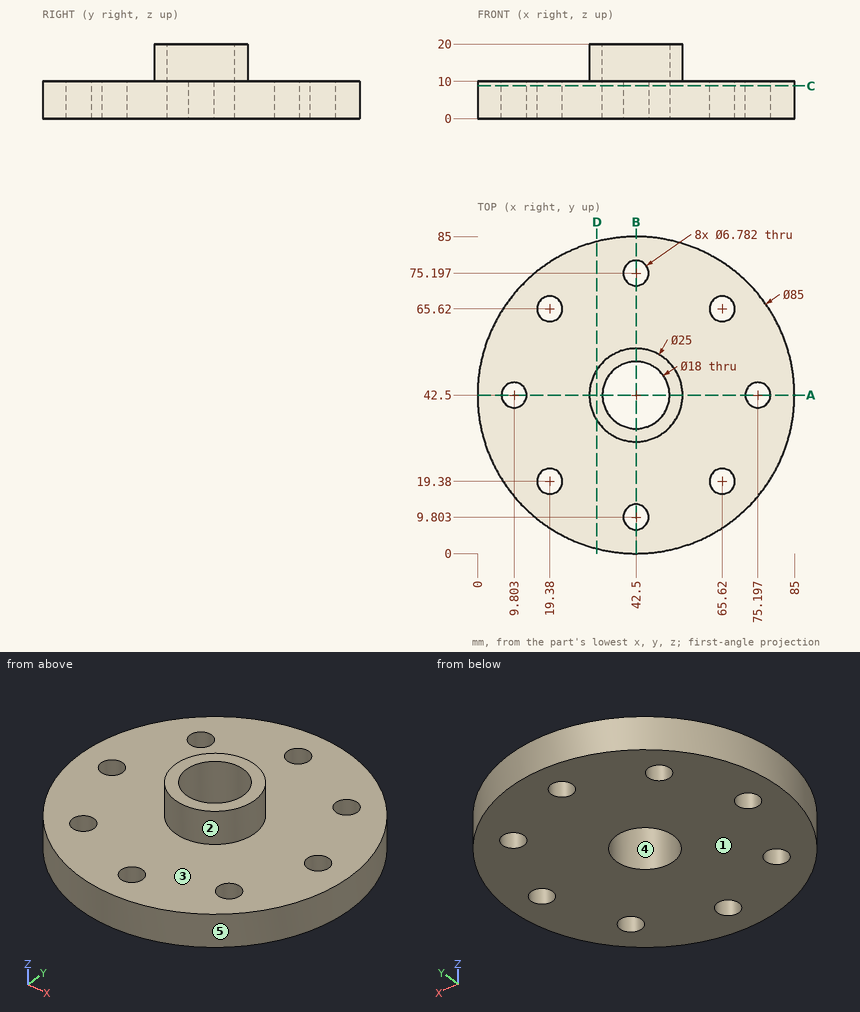
The figure shows three views and two pictorial views of one solid part (mm, origin at its lowest corner). Answer the questions. A direction names the side the tool comes from. Coordinates: 2 decimals unless noted, no trailing zeros. Loops run counter-clockwise (first coordinate to the right, second up) from the corner with the lowest first, then second, coordinate; pieces in that order, holes last. Notation, with made-up numbers: (-29.5, -1) -> (6.5, -1) arc R16 cw to (6.5, 23) -> close; hole circle Ø2 at (85, 23). An arc over 180 degrees is marked (long way). Return JSON: item names as keys, results as strings. Group by question number.
(1) Given pin 1 Ø5 at (x, y) = (16.5, 53.5) entering from +Z; pin 2 Ø1 at (x, z) = (37, 12) entering from -Y; pin 3 Ø10 at (x, z) = (75.5, 10) entering from +Y; pin 4 Ø4 at (x, y) = (19.38, 19.38) entering from -Z, each flat-ended and moving along its own axis, determine where each tip first touches the part or whether it passes through.
(2) A cutting plane is placed at D-D on x = 32. Write down the section's boundary in (y, z), and give its area (3 significant figures).
(3) Which of the six approach directions +Z, -Z, +X, -X, +Y, -Y give full straight-line access (tool end or side, diameter ignored) to the marked faces 1 and 2?
(4) A cutting plane is placed at A-A on y = 42.5. Write down the section's boundary in (x, z) (1 decimal).
(5) Find the intervals of material crossed by probe 1 along Y at (x, z) = (18, 7); probe 2 along Z at (x, y) = (16.5, 52); probe 3 along X at (y, z) = (41.5, 13.5) (1 decimal), in increasing order. Write a range as from..to.
(6) Determine the mould class of the marked faces 3, 4 and 5 for opening direction Y: released by +Y, released by -Y, zero draft, split by the parting line, or undercut.
(7) A cutting plane is placed at C-C on z = 8.75. Count the separate pieces of the cut face and the enclosed holes in it, and give its area (3 significant figures).
The answers:
{
 "1": {"pin 1": "stops at z = 10", "pin 2": "stops at y = 31.04", "pin 3": "stops at y = 74.47", "pin 4": "passes through"},
 "2": {"outline": "(1.32, 0) -> (83.68, 0) -> (83.68, 10) -> (49.28, 10) -> (49.28, 20) -> (35.72, 20) -> (35.72, 10) -> (1.32, 10) -> close", "area": "959 mm^2"},
 "3": {"face 1": "-Z, +X, -X, +Y, -Y", "face 2": "+Z"},
 "4": {"outline": "(0, 0) -> (6.4, 0) -> (6.4, 10) -> (0, 10) -> close; (13.2, 0) -> (33.5, 0) -> (33.5, 20) -> (30, 20) -> (30, 10) -> (13.2, 10) -> close; (51.5, 0) -> (71.8, 0) -> (71.8, 10) -> (55, 10) -> (55, 20) -> (51.5, 20) -> close; (78.6, 0) -> (85, 0) -> (85, 10) -> (78.6, 10) -> close"},
 "5": {"probe 1": "y = 7.77..16.28, 22.48..62.52, 68.72..77.23", "probe 2": "z = 0..10", "probe 3": "x = 30..33.6, 51.4..55"},
 "6": {"face 3": "zero draft", "face 4": "undercut", "face 5": "split by the parting line"},
 "7": {"separate pieces": "1", "enclosed holes": "9", "area": "5,130 mm^2"}
}
